Solid Edge part; units mm, degrees
sketch "Sketch1" plane through (0, 0, 0) normal (0, -1, 0) x (1, 0, 0)
  line L0 (-100, -30) -> (100, -30)
  line L1 (100, -30) -> (100, 30)
  line L2 (100, 30) -> (-100, 30)
  line L3 (-100, 30) -> (-100, -30)
  dimension "D1" = 100
  dimension "D2" = 100
extrude "Protrusion1" add sketch "Sketch1" against normal blind 2
sketch "Sketch2" plane through (0, 0, 0) normal (0, -1, 0) x (1, 0, 0)
  line L0 (-39.6222, 11.5432) -> (-48.7647, 28.7907)
  line L1 (-48.7647, 28.7907) -> (-68.9181, 28.7907)
  line L2 (-68.9181, 28.7907) -> (-78.6631, 12.1124)
  line L3 (-78.6631, 12.1124) -> (-65.8971, 12.1124)
  line L4 (-65.8971, 12.1124) -> (-62.8688, 18.0634)
  line L5 (-62.8688, 18.0634) -> (-55.6447, 18.0634)
  line L6 (-55.6447, 18.0634) -> (-51.8394, 12.1124)
  line L7 (-51.8394, 12.1124) -> (-55.6447, 5.4911)
  line L8 (-55.6447, 5.4911) -> (-62.8688, 5.4911)
  line L9 (-62.8688, 5.4911) -> (-62.8688, -5.6236)
  line L10 (-62.8688, -5.6236) -> (-55.2147, -5.6236)
  line L11 (-55.2147, -5.6236) -> (-51.8394, -11.6625)
  line L12 (-51.8394, -11.6625) -> (-55.2147, -18.0171)
  line L13 (-55.2147, -18.0171) -> (-62.8688, -18.0171)
  line L14 (-62.8688, -18.0171) -> (-65.8971, -11.6625)
  line L15 (-65.8971, -11.6625) -> (-78.6631, -11.6625)
  line L16 (-78.6631, -11.6625) -> (-68.9922, -28.7907)
  line L17 (-48.7647, -28.7907) -> (-68.9922, -28.7907)
  line L18 (-48.7647, -28.7907) -> (-39.6222, -12.3974)
  line L19 (-39.6222, -12.3974) -> (-45.6448, 0)
  line L20 (-45.6448, 0) -> (-39.6222, 11.5432)
  line L21 (-29.8239, 28.7907) -> (-39.0136, 11.3404)
  line L22 (-39.0136, 11.3404) -> (-27.2051, 11.3404)
  line L23 (-27.2051, 11.3404) -> (-23.5794, 17.7709)
  line L24 (-23.5794, 17.7709) -> (-16.2069, 17.7709)
  line L25 (-16.2069, 17.7709) -> (-12.7725, 11.3404)
  line L26 (-12.7725, 11.3404) -> (-16.2069, 5.3584)
  line L27 (-16.2069, 5.3584) -> (-23.5794, 5.3584)
  line L28 (-23.5794, 5.3584) -> (-23.5794, -5.3744)
  line L29 (-23.5794, -5.3744) -> (-16.2069, -5.3744)
  line L30 (-16.2069, -5.3744) -> (-12.7725, -11.9215)
  line L31 (-12.7725, -11.9215) -> (-16.2069, -18.0364)
  line L32 (-16.2069, -18.0364) -> (-23.5794, -18.0364)
  line L33 (-23.5794, -18.0364) -> (-27.2051, -11.9215)
  line L34 (-27.2051, -11.9215) -> (-39.0832, -11.9215)
  line L35 (-39.0832, -11.9215) -> (-39.0211, -12.3974)
  line L36 (-39.0211, -12.3974) -> (-29.8416, -28.7907)
  line L37 (-29.8416, -28.7907) -> (-9.9734, -28.7907)
  line L38 (-9.9734, -28.7907) -> (0, -11.7929)
  line L39 (0, -11.7929) -> (-6.8407, 0)
  line L40 (-6.8407, 0) -> (0, 11.8515)
  line L41 (0, 11.8515) -> (-9.9734, 28.7907)
  line L42 (-9.9734, 28.7907) -> (-29.8239, 28.7907)
  line L43 (9.4303, 28.7907) -> (0, 12.3815)
  line L44 (0, 12.3815) -> (0.2872, 11.8515)
  line L45 (0.2872, 11.8515) -> (12.5492, 11.8515)
  line L46 (12.5492, 11.8515) -> (15.7991, 18.0247)
  line L47 (15.7991, 18.0247) -> (23.265, 18.0247)
  line L48 (23.265, 18.0247) -> (26.8369, 11.8515)
  line L49 (26.8369, 11.8515) -> (23.265, 5.318)
  line L50 (23.265, 5.318) -> (15.7991, 5.318)
  line L51 (15.7991, 5.318) -> (15.7991, -5.632)
  line L52 (15.7991, -5.632) -> (23.265, -5.632)
  line L53 (23.265, -5.632) -> (26.7839, -11.7003)
  line L54 (26.7839, -11.7003) -> (23.265, -17.8487)
  line L55 (23.265, -17.8487) -> (15.768, -17.8487)
  line L56 (15.768, -17.8487) -> (12.2913, -11.7003)
  line L57 (0.3007, -11.6312) -> (12.2913, -11.7003)
  line L58 (0, -12.7084) -> (0.3007, -11.6312)
  line L59 (0, -12.7084) -> (9.391, -28.7907)
  line L60 (9.391, -28.7907) -> (29.5768, -28.7907)
  line L61 (29.5768, -28.7907) -> (39.4696, -11.7929)
  line L62 (39.4696, -11.7929) -> (32.5504, 0)
  line L63 (39.014, 12.1809) -> (32.5504, 0)
  line L64 (29.5768, 28.7907) -> (39.014, 12.1809)
  line L65 (29.5768, 28.7907) -> (9.4303, 28.7907)
  line L66 (39.3531, 11.3913) -> (49.0927, 28.7907)
  line L67 (68.964, 28.7907) -> (49.0927, 28.7907)
  line L68 (78.6631, 11.3946) -> (68.964, 28.7907)
  line L69 (55.3829, -28.7907) -> (78.6631, 11.3946)
  line L70 (42.8739, -28.7907) -> (55.3829, -28.7907)
  line L71 (56.0977, -5.4746) -> (42.8739, -28.7907)
  line L72 (49.0927, -5.4746) -> (56.0977, -5.4746)
  line L73 (49.0927, -5.4746) -> (39.3531, 11.3913)
  line L74 (51.7218, 11.7746) -> (55.3868, 5.6144)
  line L75 (55.3868, 5.6144) -> (62.6387, 5.6144)
  line L76 (62.6387, 5.6144) -> (66.3037, 11.7746)
  line L77 (66.3037, 11.7746) -> (62.6387, 17.9349)
  line L78 (62.6387, 17.9349) -> (55.3868, 17.9349)
  line L79 (55.3868, 17.9349) -> (51.7218, 11.7746)
extrude "ExtrudedProtrusion_3" add sketch "Sketch2" along normal blind 3
sketch "Sketch3" plane through (0, 0, 0) normal (0, -1, 0) x (1, 0, 0)
  line L0 (0, -30) -> (0, 30)
  line L1 (0, 30) -> (100, 30)
  line L2 (100, 30) -> (100, -30)
  line L3 (100, -30) -> (0, -30)
  line L4 (-78.6631, 30) -> (-78.6631, -30)
  line L5 (-78.6631, -30) -> (-100, -30)
  line L6 (-100, -30) -> (-100, 30)
  line L7 (-100, 30) -> (-78.6631, 30)
extrude "ExtrudedCutout_1" cut sketch "Sketch3" along normal blind 14.3776
sketch "Sketch4" plane through (0, 0, 0) normal (0, -1, 0) x (1, 0, 0)
  line L0 (0, 30) -> (100, 30)
  line L1 (100, 30) -> (100, -30)
  line L2 (100, -30) -> (0, -30)
  line L3 (0, -30) -> (0, 30)
  line L4 (-100, 30) -> (-78.6631, 30)
  line L5 (-78.6631, 30) -> (-78.6631, -30)
  line L6 (-78.6631, -30) -> (-100, -30)
  line L7 (-100, -30) -> (-100, 30)
extrude "ExtrudedCutout_2" cut sketch "Sketch4" against normal blind 57.8718
properties part number "BumbleB0911"
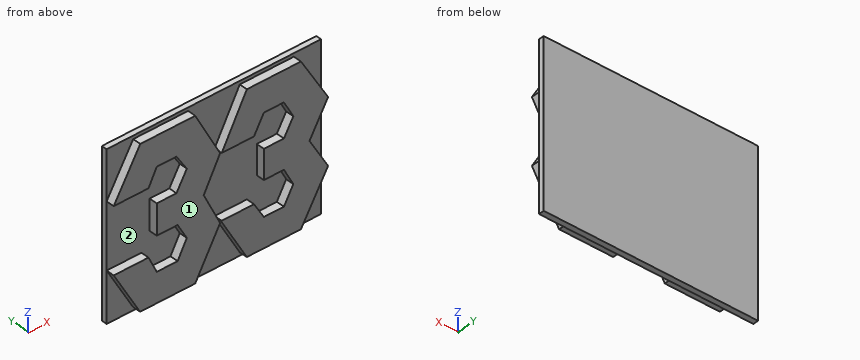
CAD build for the part. Positions are in the model's coordinates, mm. Face numbers are marked on the shaded views. Coordinates: 2 decimals unless noted, no trailing zeros. Order: outer loops, then holes, each group sorted by start corner. A loop starts at its lowest first (then second) coordinate and runs counter-clockwise, first axis right, second up. Notation, with made-up numbers: M 51.25,-15 L 109.25,-15 A26 cw 109.25,16 Z; hole C -6,6.25 d9. An arc over 180 degrees is marked long. Write each question's results on one line, items separated by ' | '. Start each with the question number.
Q1. Flat gauge pins, fed straight in: P1, Ø1.5, axis at x = -24, y = -1.5, coming from the -Z side; P2, Ø2.5, axis at y = -2, z = 1, coming from the -X side; P3, Ø2.5, axis at x = -74, y = -2, coming from the +Z side. Where does each tip first touch, or does it go through?
Q2. Cut at C-C (z = -23.5). List the corners of the cut face in (x, y).
Q3. Cut at D-D (x = -47.5). List the corners of the cut face in (y, z).
Q4. Cut at B-B (z = 1). List the corners of the cut face in (x, y), then the cut area to 3 significant figures.
Q5. Drill centre lines: probe 1 along Z at (x, y) = (-23, -0.1); probe 2 along X at (y, z) = (-0.9, -17); probe 3 along Y at (x, z) = (-21.5, -16.5). Where is each one in solid material? Low to high. Write a range as from..to.
Q6. Pull direction X, two halves, no side cores. Call the marked faces 1 and 2: +X half, -X half, draft (parallel to the pull), parting line (faces both ways), or undercut.
Q7. Cut at A-A (x = -60.5). List the corners of the cut face in (y, z).
Found:
1) P1: z = -28.79 | P2: x = -62.87 | P3: z = 22.23
2) outline: M -78.66,0 L -71.98,0 L -71.98,-3 L -45.81,-3 L -45.81,0 L -32.8,0 L -32.8,-3 L -6.87,-3 L -6.87,0 L 0,0 L 0,2 L -78.66,2 Z
3) outline: M -3,-26.52 L 0,-26.52 L 0,-30 L 2,-30 L 2,30 L 0,30 L 0,26.4 L -3,26.4 Z
4) outline: M -78.66,0 L -62.87,0 L -62.87,-3 L -45.12,-3 L -45.12,0 L -23.58,0 L -23.58,-3 L -6.26,-3 L -6.26,0 L 0,0 L 0,2 L -78.66,2 Z | area: 263 mm²
5) probe 1: -28.79..-18.04, -5.37..5.36, 17.77..28.79 | probe 2: -75.65..-63.35, -54.67..-42.19, -36.44..-24.19, -15.62..-3.06 | probe 3: 0..2
6) face 1: draft | face 2: undercut
7) outline: M -3,-28.79 L 0,-28.79 L 0,-30 L 2,-30 L 2,30 L 0,30 L 0,28.79 L -3,28.79 L -3,18.06 L 0,18.06 L 0,5.49 L -3,5.49 L -3,-5.62 L 0,-5.62 L 0,-18.02 L -3,-18.02 Z
